Can you work these out from the drawing? Everything is in mm from the part's minimum corner. A direction names the side the tool comes from. Coordinates: 2 decimals unless noted, no trailing zeros. Order: outer loops, then holes, each group sorted by start corner. A loop starts at its lowest first (then second) coordinate and runs counter-clockwise, first axis right, second up. Notation, with made-up numbers: M 58,81 L 117,81 A24 cw 117,113 Z; hole C 84,46.25 d3. An arc over 180 degrees is marked long. One line per question, with ' | ' between items. Start each with the question number.
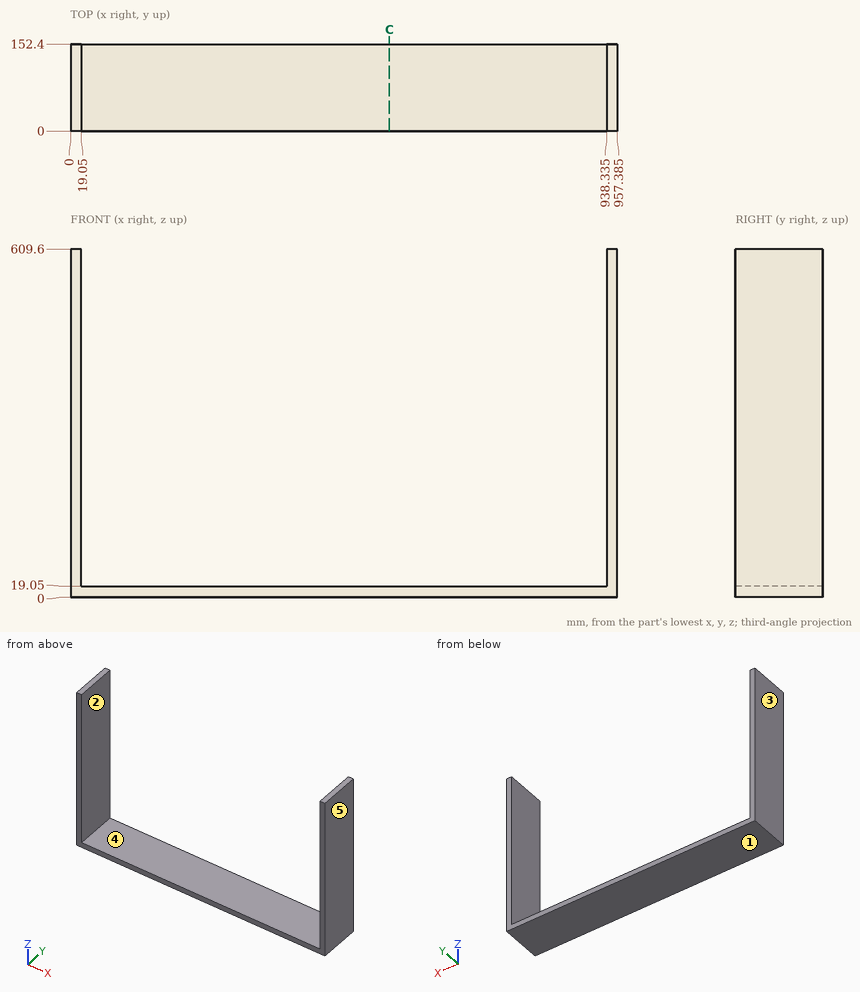
(1) We'd pull the mould along X, two halves only. Please class the marked faces 1, 2 and 3: +X half, -X half, draft (parallel to the pull), parting line (faces both ways), or undercut.
(2) Imagine slicing it at C-C, the plane x = 558. Write out the boundary of the cut face in (y, z).
(3) On a 3-axis mill with a long thin cutter (end or side, diameter ignored), from which of +Z, -Z, +X, -X, +Y, -Y can I reach the whole of each face in a straight line? I mean the marked faces 4 and 5. Say none if no direction works.
(4) If I drill on line 1 along Z through (x, y) = (198.5, 51), over which ranges is the centre line in solid material (lowest first)? Write a range as from..to.
(5) For P1, Ø4, axis at x = 115.5, y = 132.5, coming from the +Z side; P2, Ø8, axis at x = 321, y = 127.5, coming from the -Z side, each with a flat end and sliding along its axis, tell me the tip position at first contact or that it passes through.
Answers:
1) face 1: draft | face 2: undercut | face 3: -X half
2) outline: M 0,0 L 152.4,0 L 152.4,19.05 L 0,19.05 Z
3) face 4: +Z, +Y, -Y | face 5: +Z, -Z, +X, +Y, -Y
4) line 1: 0..19.05
5) P1: z = 19.05 | P2: z = 0
